For this review, take the finished solid that the model builds, in its own axes (mm). A direction names the side the tool comes from. Round coordinates to 2 decimals unless told otherwise and drop trailing zeros. Order: outer loops, then holes, each group sorted by start corner. A loop starts at its lowest first (then second) coordinate and runs counter-clockwise, first axis right, second up. Notation, with made-up numbers: M -9.5,-11 L 46.5,-11 A21 ccw 46.5,17 Z; hole C 62.25,3 d2. An arc over 180 degrees is marked long. Answer as a JSON object with one key per item and string values.
from build123d import *

# Parameters (mm, degrees)
F0_R          = 1.95
F1_DEPTH      = 0.8
F2_R          = 1.5
F3_DEPTH      = 4.5
F4_R          = 1.5
F6_DEPTH      = 0.25
F6_DEPTH_BACK = 0.25


with BuildPart() as f1:
    # F0 (on Top) → F1 (new body)
    with BuildSketch(Plane.XY):
        Circle(F0_R)
    extrude(amount=F1_DEPTH)

    # F2 (on face) → F3 (join)
    with BuildSketch(Plane.XY.offset(0.8)):
        Circle(F2_R)
    extrude(amount=F3_DEPTH)

    # F4
    f4_edges = [f1.edges().sort_by_distance(p)[0] for p in [
        (-1.5, 0, 5.3),
    ]]
    fillet(f4_edges, radius=F4_R)

    # F5 (on Front) → F6 (join, two sides)
    with BuildSketch(Plane.XZ) as f6_sk:
        Polygon((-2.29, -1.340597), (-2.54, -1.623856), (-2.54, -7.528054), (-2.29, -7.528054), (-2.29, -2.096204), align=None)
        Polygon((-2.54, -7.528054), (-2.54, -1.623856), (-2.79, -1.907115), (-2.79, -7.528054), align=None)
        Polygon((-1.106809, 0), (-2.29, -1.340597), (-2.29, -2.096204), (-0.731933, -0.33086), (-0.25, -0.33086), (0.25, -0.33086), (0.731933, -0.33086), (2.29, -2.096204), (2.29, -1.340597), (1.106809, 0), align=None)
        Polygon((0.25, -0.33086), (-0.25, -0.33086), (-0.25, -7.528054), (0, -7.528054), (0.25, -7.528054), align=None)
        Polygon((2.54, -1.623856), (2.29, -1.340597), (2.29, -2.096204), (2.29, -7.528054), (2.54, -7.528054), align=None)
        Polygon((2.79, -1.907115), (2.54, -1.623856), (2.54, -7.528054), (2.79, -7.528054), align=None)
    extrude(amount=F6_DEPTH)
    extrude(f6_sk.sketch, amount=-F6_DEPTH_BACK)


solid = f1.part
1) Add section C-C on y = 0. State the section outline as (x, z) points.
Geometry check:
{"outline": "M -2.79,-7.53 L -2.29,-7.53 L -2.29,-2.1 L -0.73,-0.33 L -0.25,-0.33 L -0.25,-7.53 L 0.25,-7.53 L 0.25,-0.33 L 0.73,-0.33 L 2.29,-2.1 L 2.29,-7.53 L 2.79,-7.53 L 2.79,-1.91 L 2.29,-1.34 L 1.11,0 L 1.95,0 L 1.95,0.8 L 1.5,0.8 L 1.5,3.8 A1.5 ccw -1.5,3.8 L -1.5,0.8 L -1.95,0.8 L -1.95,0 L -1.11,0 L -2.29,-1.34 L -2.79,-1.91 Z"}
2) Machinability: for faces 1 (the cylindrical face through (-1.5, 0.07, 2.28)), 2 (the flat face through (1.5, 0, -1.2)), 3 (the flat face through (0, 0.25, -3)), 4 (the flat face through (0, -0.25, -3)), which of the approach directions +Z, -Z, +X, -X, +Y, -Y give a long, thin tool a straight path to every point of the face, cutting with its end or side? Answer none if there is none.
Geometry check:
{"face 1": "+Z", "face 2": "-Z, +Y, -Y", "face 3": "-Z, +X, -X, +Y", "face 4": "-Z, +X, -X, -Y"}
3) Add section B-B on x = 0. State the section outline as (y, z) points.
Geometry check:
{"outline": "M -1.95,0 L -0.25,0 L -0.25,-7.53 L 0.25,-7.53 L 0.25,0 L 1.95,0 L 1.95,0.8 L 1.5,0.8 L 1.5,3.8 A1.5 ccw -1.5,3.8 L -1.5,0.8 L -1.95,0.8 Z"}
4) For L1, parallel to X at y = 0.2, z = -4.75; L2, parallel to Z at x = 0.45, y = 1.65; L3, parallel to Z at x = 1.65, y = 0, list the stretches that pass through material, from the lowest coordinate up.
Geometry check:
{"L1": "x = -2.79 to -2.29, -0.25 to 0.25, 2.29 to 2.79", "L2": "z = 0 to 0.8", "L3": "z = -1.37 to -0.62, 0 to 0.8"}
5) Add section D-D on y = -1.05. State the section outline as (x, z) points.
Geometry check:
{"outline": "M -1.64,0 L 1.64,0 L 1.64,0.8 L 1.07,0.8 L 1.07,3.8 A1.07 ccw -1.07,3.8 L -1.07,0.8 L -1.64,0.8 Z"}
6) Insertion check: P1, Ø1.5, axis at x = 1.5, z = 1, coming from the +Y side; P2, Ø2, axis at x = 1, y = -1.5, coming from the -Z side; P3, Ø1.7, axis at x = 0.5, z = -2, coming from the +Y side. Each pin has a flat end and moves straight along its axis. Give the tip position at first contact, or say it passes through.
Geometry check:
{"P1": "stops at y = 1.79", "P2": "stops at z = 0", "P3": "stops at y = 0.25"}
7) Add section A-A on z = -2.5. State the section outline as (x, y) points.
Geometry check:
{"outline": "M -2.79,-0.25 L -2.29,-0.25 L -2.29,0.25 L -2.79,0.25 Z; M -0.25,-0.25 L 0.25,-0.25 L 0.25,0.25 L -0.25,0.25 Z; M 2.29,-0.25 L 2.79,-0.25 L 2.79,0.25 L 2.29,0.25 Z"}
